Part model, mm, in its own coordinate system. A direction names the side the tool comes from. Coordinates: 2 decimals unless noted, no trailing zeros. Write each loop counter-clockwise with the first axis right and the second up, starting at its lowest first coordinate (ties: lowest second). Pieces come first, ordered by that corner, then holes. Notation, with made-up numbers: (85.25, 58.5) -> (90.25, 58.5) arc R15 ccw to (90.25, 87.5) -> close; hole circle Ø2 at (38.25, 75). An arc over 180 degrees is marked (long way). Write item = value, one per line. Start each with the question number.
Q1. Band-saw the part on A-A, the plane y = 55. List the corners of the cut face in (x, z), plus the area to 3 significant figures.
Q2. Pull direction Y, two halves, no side cores. Call faces 1 (the flat face through (-10, 65, -4)), 2 (the flat face through (-48, 48, 0)), 3 (the cylindrical face through (33.4, 55.07, -3.73)), 4 (the flat face through (-21, 60, 3)): released by +Y, released by -Y, zero draft, split by the parting line, or undercut.
Q3. Band-saw the part on B-B, the plane y = -30. List the corners of the cut face in (x, z).
Q4. Tool access for faces 5 (the flat face through (-20, 55, 0)), 6 (the cylindrical face through (9, 46.57, -0.07)), 7 (the flat face through (30, 55, -2.5)): list every direction of +Z, -Z, +X, -X, +Y, -Y with a clear straight run to the whole face (end or side of a thin tool).
Q5. Probe line 1 (Z direction, x = -0.25, y = -30); line 2 (Y direction, x = 43.5, z = -2.5); line 3 (X direction, y = 20.5, z = -1). List the from-to ranges inside material, lowest first.
Q6. Pin check, flat tips, straight feed: P1, Ø3, axis at y = -13.5, z = 2, coming from the +X side; P2, Ø1.5, axis at x = 25, z = -2.5, coming from the +Y side; P3, Ø4, axis at y = -30, z = 0, coming from the -X side. Stop position of each tip, or through.
Q7. Band-saw the part on C-C, the plane x = 6. List the corners of the cut face in (y, z).
Q8. Band-saw the part on D-D, the plane x = 50.5. List the corners of the cut face in (y, z).
from build123d import *

# Parameters (mm, degrees)
F0_W      = 15
F0_H      = 100
F1_DEPTH  = 5
F2_W      = 80
F2_H      = 10
F3_DEPTH  = 10
F4_W      = 10
F4_H      = 5
F5_DEPTH  = 20
F6_W      = 10
F6_H      = 5
F7_DEPTH  = 20
F8_R      = 1.6
F9_DEPTH  = 10
F10_W     = 67.5
F10_H     = 10
F10_W_2   = 120
F11_DEPTH = 2
F12_R     = 5
F13_R     = 1.6
F14_DEPTH = 15
F15_W     = 20
F15_H     = 10
F16_DEPTH = 5
F17_W     = 20
F17_H     = 6.5
F18_DEPTH = 3
F19_DEPTH = 10
F21_DEPTH = 10


# Not quite as in the source:
# - a pattern or mirror of a feature is missing from the dataset's text; its kind, count and spacing are read off the source's solid


with BuildPart() as f1:
    # F0 (on Top) → F1 (new body, symmetric)
    with BuildSketch(Plane.XY):
        Rectangle(F0_W, F0_H)
    extrude(amount=F1_DEPTH, both=True)

    # F2 (on face) → F3 (join)
    with BuildSketch(Plane(origin=(0, 50, 0), x_dir=(-1, 0, 0), z_dir=(0, 1, 0))):
        Rectangle(F2_W, F2_H)
    extrude(amount=F3_DEPTH)

    # F4 (on face) → F5 (cut)
    with BuildSketch(Plane(origin=(-40, 0, 0), x_dir=(0, -1, 0), z_dir=(-1, 0, 0))):
        with Locations((-55, 0)):
            Rectangle(F4_W, F4_H)
    extrude(amount=-F5_DEPTH, mode=Mode.SUBTRACT)

    # F6 (on face) → F7 (cut)
    with BuildSketch(Plane.YZ.offset(40)):
        with Locations((55, 0)):
            Rectangle(F6_W, F6_H)
    extrude(amount=-F7_DEPTH, mode=Mode.SUBTRACT)

    # F8 (on face) → F9 (cut, through all)
    with BuildSketch(Plane.XY.offset(5)):
        with Locations((-35, 55)):
            Circle(F8_R)
        with Locations((35, 55)):
            Circle(F8_R)
    extrude(amount=-F9_DEPTH, mode=Mode.SUBTRACT)

    # F10 (on face) → F11 (join)
    with BuildSketch(Plane.XZ.offset(-50)):
        with Locations((26.25, 0)):
            Rectangle(F10_W, F10_H)
        Rectangle(F10_W_2, F10_H)
    extrude(amount=F11_DEPTH)

    # F12
    f12_edges = [f1.edges().sort_by_distance(p)[0] for p in [
        (-7.5, 48, 0),
        (7.5, 48, 0),
    ]]
    fillet(f12_edges, radius=F12_R)

    # F13 (on face) → F14 (cut, through all)
    with BuildSketch(Plane(origin=(-7.5, 0, 0), x_dir=(0, -1, 0), z_dir=(-1, 0, 0))):
        with Locations((30, 0)):
            Circle(F13_R)
        with Locations((45, 0)):
            Circle(F13_R)
    extrude(amount=-F14_DEPTH, mode=Mode.SUBTRACT)

    # F15 (on face) → F16 (join)
    with BuildSketch(Plane(origin=(0, 60, 0), x_dir=(-1, 0, 0), z_dir=(0, 1, 0))):
        Rectangle(F15_W, F15_H)
    extrude(amount=F16_DEPTH)

    # F17 (on face) → F18 (cut)
    with BuildSketch(Plane(origin=(0, 65, 0), x_dir=(-1, 0, 0), z_dir=(0, 1, 0))):
        Rectangle(F17_W, F17_H)
    extrude(amount=-F18_DEPTH, mode=Mode.SUBTRACT)

    # F19 (add): a face of the model
    f19_faces = [f1.faces().sort_by_distance(p)[0] for p in [
        (0, 65, -4.125),
    ]]
    extrude(f19_faces, amount=F19_DEPTH)

    # F20 (on face) → F21 (join, through all)
    with BuildSketch(Plane.XY.offset(5)):
        with BuildLine():
            Line((35, 48), (30, 48))
            ThreePointArc((30, 48), (23.7170824513, 29.6288269291), (7.5, 18.9526249034))
            Line((7.5, 18.9526249034), (7.5, 13.8130141721))
            ThreePointArc((7.5, 13.8130141721), (27.2717802866, 26.0625890315), (35, 48))
        make_face()
    f21 = extrude(amount=-F21_DEPTH)

    # F21_copies: F21 across plane
    add(f21.mirror(Plane(origin=(0, 0, 0), x_dir=(0, 0, -1), z_dir=(-1, 0, 0))))


solid = f1.part
Ans:
q1.outline = (-40, -5) -> (-36.6, -5) -> (-36.6, -2.5) -> (-40, -2.5) -> close; (-40, 2.5) -> (-36.6, 2.5) -> (-36.6, 5) -> (-40, 5) -> close; (-33.4, -5) -> (33.4, -5) -> (33.4, -2.5) -> (20, -2.5) -> (20, 2.5) -> (33.4, 2.5) -> (33.4, 5) -> (-33.4, 5) -> (-33.4, 2.5) -> (-20, 2.5) -> (-20, -2.5) -> (-33.4, -2.5) -> close; (36.6, -5) -> (40, -5) -> (40, -2.5) -> (36.6, -2.5) -> close; (36.6, 2.5) -> (40, 2.5) -> (40, 5) -> (36.6, 5) -> close
q1.area = 568 mm2
q2.face_1 = zero draft
q2.face_2 = released by -Y
q2.face_3 = undercut
q2.face_4 = released by +Y
q3.outline = (-7.5, -5) -> (7.5, -5) -> (7.5, -1.6) -> (-7.5, -1.6) -> close; (-7.5, 1.6) -> (7.5, 1.6) -> (7.5, 5) -> (-7.5, 5) -> close
q4.face_5 = -X, +Y
q4.face_6 = +Z, -Z
q4.face_7 = +X, +Y
q5.line_1 = -5 to -1.6, 1.6 to 5
q5.line_2 = 48 to 50
q5.line_3 = -21.65 to -11.99, -7.5 to 7.5, 11.99 to 21.65
q6.P1 = 7.5
q6.P2 = 60
q6.P3 = -7.5
q7.outline = (-50, -5) -> (75, -5) -> (75, -3.25) -> (62, -3.25) -> (62, 3.25) -> (65, 3.25) -> (65, 5) -> (-50, 5) -> close; hole circle Ø3.2 at (-45, 0); hole circle Ø3.2 at (-30, 0)
q8.outline = (48, -5) -> (50, -5) -> (50, 5) -> (48, 5) -> close
